Geometry: final body of the model. Coordinates: model frame, mm. A direction names the side the tool comes from. Coordinates: 2 decimals unless noted, no trailing zeros. Write each loop counter-clockwise with the first axis right and the second up, starting at its lowest first coordinate (ties: lowest second). Pieces come first, ordered by that corner, then holes. Notation, with made-up numbers: (-14.75, -1) - (40.25, -1) arc R19 ccw to (40.25, 30) - close; hole circle Ø7 at (67.25, 37). An arc over 180 degrees is marked (long way). Answer as a JSON object with one key per item and string values. Group by question number.
Item 1: First-contact query: pin 1 Ø1 at (x, z) = (47.5, 1017.5) entering from -Y; pin 2 Ø10 at (y, z) = (102, 503) entering from -X; pin 3 Ø3 at (y, z) = (-124.5, 1687.5) entering from +X. Flat tips, straight axial feed; report the tip coordinate or a pass-through.
Item 2: Line query: line 1 along Z through (x, y) = (264, -67); line 2 along Z through (x, y) = (-425, 275.5); line 3 along Y through (x, z) = (-7, 819). Output: solid intervals per line, ascending. Write a range as from..to.
Item 3: Set-up query: faces 1 (the flat face through (-351.477, 3, 379)), 2 (the flat face through (273, -273, 254)), 3 (the flat face through (173.278, -305.808, 379.222)), 4 (the flat face through (178.199, 302.967, 379.222)), 5 (the flat face through (-173.278, 305.808, 1903.222)). Return all of +Z, -Z, +X, -X, +Y, -Y with unobstructed straight access to the full face (end or side cutting, diameter ignored); none if empty.
Item 4: Section B-B on y = 261.5. Return loops of the section in (x, z), and give its area (3 significant figures).
Item 5: Section A-A on x = -254. Return loops of the section in (y, z), and give its area (3 significant figures).
Item 6: Section C-C on z = 339.5. Return loops of the section in (x, y).
Item 7: Mould query, pull axis Z, two halves, no side actions, for faces 6 (the flat face through (-351.477, 3, 1903)), 7 (the flat face through (-2, 2, 2286)), 8 (the flat face through (-161, -85, 508)). Classes: pulls with the +Z half, pulls with the -Z half, needs draft (parallel to the pull), parting line crosses it, or undercut.
Item 8: Section D-D on y = 0. Return loops of the section in (x, z), and give its area (3 significant figures).
```python
from build123d import *

# Parameters (mm, degrees)
F0_R      = 635
F1_DEPTH  = 254
F3_DEPTH  = 254
F4_R      = 177.5274912945
F5_DEPTH  = 1778
F6_START  = 1270
F3_FACE_R = 177.5274912945
F6_DEPTH  = 254


with BuildPart() as f1:
    # F0 (on Top) → F1 (new body)
    with BuildSketch(Plane.XY):
        Circle(F0_R)
    extrude(amount=F1_DEPTH)

    # F2 (on face) → F3 (join)
    with BuildSketch(Plane.XY.offset(254)):
        Polygon((351.4767885208, -202.9252184664), (351.4767885208, 202.9252184664), (0, 405.8504369328), (-351.4767885208, 202.9252184664), (-351.4767885208, -202.9252184664), (0, -405.8504369328), align=None)
    extrude(amount=F3_DEPTH)

    # F4 (on face) → F5 (join)
    with BuildSketch(Plane.XY.offset(508)):
        Circle(F4_R)
    extrude(amount=F5_DEPTH)

    # F3_face (on face) → F6 (join)
    with BuildSketch(Plane.XY.offset(508).offset(F6_START)):
        Polygon((0, -405.8504369328), (351.4767885208, -202.9252184664), (351.4767885208, 202.9252184664), (0, 405.8504369328), (-351.4767885208, 202.9252184664), (-351.4767885208, -202.9252184664), align=None)
        Circle(F3_FACE_R, mode=Mode.SUBTRACT)
    extrude(amount=F6_DEPTH)


solid = f1.part
```
Checks:
{
 "1": {"pin 1": "y = -171.19", "pin 2": "x = -351.48", "pin 3": "x = 128.01"},
 "2": {"line 1": "0..508, 1778..2032", "line 2": "0..254", "line 3": "-177.39..177.39"},
 "3": {"face 1": "+Z, -X, +Y, -Y", "face 2": "+Z", "face 3": "+Z, +X, -Y", "face 4": "+Z, +X, +Y", "face 5": "+Z, -X, +Y"},
 "4": {"outline": "(-578.66, 0) - (578.66, 0) - (578.66, 254) - (250.02, 254) - (250.02, 508) - (-250.02, 508) - (-250.02, 254) - (-578.66, 254) - close; (-250.02, 1778) - (250.02, 1778) - (250.02, 2032) - (-250.02, 2032) - close", "area": "548,000 mm^2"},
 "5": {"outline": "(-581.99, 0) - (581.99, 0) - (581.99, 254) - (259.2, 254) - (259.2, 508) - (-259.2, 508) - (-259.2, 254) - (-581.99, 254) - close; (-259.2, 1778) - (259.2, 1778) - (259.2, 2032) - (-259.2, 2032) - close", "area": "559,000 mm^2"},
 "6": {"outline": "(-351.48, -202.93) - (0, -405.85) - (351.48, -202.93) - (351.48, 202.93) - (0, 405.85) - (-351.48, 202.93) - close"},
 "7": {"face 6": "needs draft", "face 7": "pulls with the +Z half", "face 8": "undercut"},
 "8": {"outline": "(-635, 0) - (635, 0) - (635, 254) - (351.48, 254) - (351.48, 508) - (177.53, 508) - (177.53, 1778) - (351.48, 1778) - (351.48, 2032) - (177.53, 2032) - (177.53, 2286) - (-177.53, 2286) - (-177.53, 2032) - (-351.48, 2032) - (-351.48, 1778) - (-177.53, 1778) - (-177.53, 508) - (-351.48, 508) - (-351.48, 254) - (-635, 254) - close", "area": "1,220,000 mm^2"}
}
